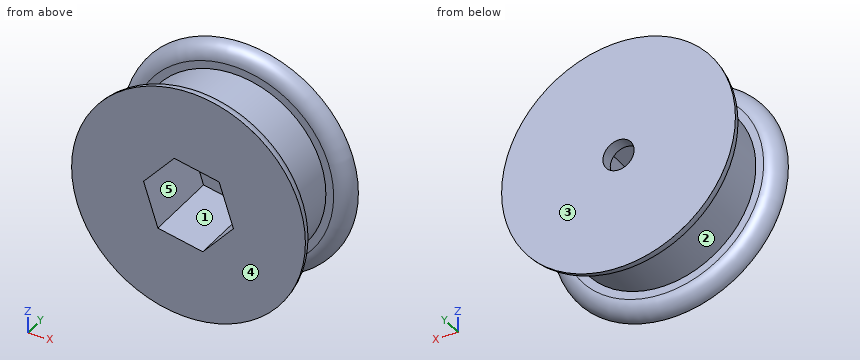
Autodesk Inventor part; units mm, degrees
ref_plane "YZ Plane" through (0, 0, 0) normal (1, 0, 0) x (0, 1, 0)
ref_plane "XZ Plane" through (0, 0, 0) normal (0, 1, 0) x (-1, 0, 0)
ref_plane "XY Plane" through (0, 0, 0) normal (0, 0, 1) x (1, 0, 0)
sketch "스케치1" plane through (0, 0, 0) normal (0, 1, 0) x (-1, 0, 0)
  line L0 (-0.9169, -2.7981) -> (-2.8817, -0.6049)
  line L1 (-2.8817, -0.6049) -> (-1.9647, 2.1931)
  line L2 (-1.9647, 2.1931) -> (0.9169, 2.7981)
  line L3 (0.9169, 2.7981) -> (2.8817, 0.6049)
  line L4 (2.8817, 0.6049) -> (1.9647, -2.1931)
  line L5 (1.9647, -2.1931) -> (-0.9169, -2.7981)
  circle A0 centre (0, 0) radius 7.5
  dimension "d0" = 5.1
  dimension "d1" = 15
extrude "돌출1" add sketch "스케치1" along normal blind 1
sketch "스케치2" plane through (0, 1, 0) normal (0, 1, 0) x (1, 0, 0)
  circle A0 centre (0, 0) radius 6
  line L0 (2.8817, 0.6049) -> (1.9647, -2.1931)
  line L1 (1.9647, -2.1931) -> (-0.9169, -2.7981)
  line L2 (-0.9169, -2.7981) -> (-2.8817, -0.6049)
  line L3 (-2.8817, -0.6049) -> (-1.9647, 2.1931)
  line L4 (-1.9647, 2.1931) -> (0.9169, 2.7981)
  line L5 (0.9169, 2.7981) -> (2.8817, 0.6049)
  circle A1 centre (0, 0) radius 7.5
  dimension "d4" = 12
extrude "돌출2" add sketch "스케치2" along normal blind 3.8 contours A0
sketch "스케치3" plane through (0, 4.8, 0) normal (0, 1, 0) x (1, 0, 0)
  circle A0 centre (0, 0) radius 7.5
  circle A1 centre (0, 0) radius 7.5
  line L0 (1.9647, -2.1931) -> (-0.9169, -2.7981)
  line L1 (-0.9169, -2.7981) -> (-2.8817, -0.6049)
  line L2 (-2.8817, -0.6049) -> (-1.9647, 2.1931)
  line L3 (-1.9647, 2.1931) -> (0.9169, 2.7981)
  line L4 (0.9169, 2.7981) -> (2.8817, 0.6049)
  line L5 (2.8817, 0.6049) -> (1.9647, -2.1931)
  circle A2 centre (0, 0) radius 6
  dimension "d7" = 15
extrude "돌출3" add sketch "스케치3" along normal blind 1 contours A0 | A2
sketch "스케치4" plane through (0, 5.8, 0) normal (0, 1, 0) x (1, 0, 0)
  point P0 (0, 0)
sketch "스케치5" plane through (0, 5.8, 0) normal (0, 1, 0) x (1, 0, 0)
  circle A0 centre (0, 0) radius 5
  circle A1 centre (0, 0) radius 1
  dimension "d10" = 10
  dimension "d11" = 2
extrude "돌출4" add sketch "스케치5" against normal blind 0.8
fillet "모깎기1" radius 1 2 edges at (7.5, 1, 0) (-7.5, 4.8, 0)
sketch "스케치6" plane through (0.9169, 0, -2.7981) normal (-0.7448, 0, 0.6673) x (0.6673, 0, 0.7448)
  point P0 (1.4722, 0)
sketch "스케치7" plane through (-2.8817, 0, 0.6049) normal (0.9503, 0, 0.3114) x (0.3114, 0, -0.9503)
  point P0 (1.4722, 0)
properties part number "motor gear"
Work out the finished part from the listing and answer in its coordinate system (mm). Face numbers are marked on the shaded views. A direction names the side the tool comes from. Round coordinates to 2 decimals unless told otherwise and drop trailing zeros. Order: outer loops, then holes, each group sorted by start corner. A loop starts at its lowest first (then second) coordinate and runs counter-clockwise, first axis right, second up. Notation, with made-up numbers: M 73.5,-4 L 100.5,-4 A15 cw 100.5,5 Z; hole C 17,25.5 d1. An arc over 180 degrees is marked long. Put each result on its own line as item: value. Start each with the question number.
Q1. Flat-ended cylindrical pins translate along their axes: pin 1 (3 mm diameter, centred on x = -2.5, y = 3, fed in from -Z); pin 2 (2 mm diameter, centred on x = 0, y = 2.5, fed in from +Z); pin 3 (4 mm diameter, centred on x = 0, z = 0.5, fed in from -Y). Find the tip coordinate at first contact, or state that the pin passes through.
Q2. Straight lines are drawn through the part: L1, parallel to Y at x = -6, z = 1.25; L2, parallel to X at y = 2, z = 1; L3, parallel to Y at x = -1.25, z = -1.5. For each, find the intervals that lie inside material, in ascending order. Write a range as [from, to].
Q3. Section A-A, the plane y = 2.1 is taken. Write down the section's boundary in (x, z), and give its area (3 significant figures).
Q4. For a pull along X with two mould halves and no side action, classify the marked faces 1, 2 and 3 as pulls with the +X half, pulls with the -X half, needs draft (parallel to the pull), parting line crosses it, or undercut.
Q5. A tool of negligible diameter and unlimited length cuts with its end or side. For the marked faces 4 and 5, from which of +Z, -Z, +X, -X, +Y, -Y can it reach the whole face along a straight path? Write none if from no direction.
Findings below:
1. pin 1: stops at z = -5.92
1. pin 2: stops at z = 6
1. pin 3: stops at y = 5
2. L1: y = [0, 1], [4.8, 5.8]
2. L2: x = [-5.92, -2.53], [2.36, 5.92]
2. L3: y = [5, 5.8]
3. outline: C 0,0 d12; hole M -2.88,0.6 L -1.96,-2.19 L 0.92,-2.8 L 2.88,-0.6 L 1.96,2.19 L -0.92,2.8 Z
3. area: 90.6 mm^2
4. face 1: undercut
4. face 2: parting line crosses it
4. face 3: needs draft
5. face 4: +Z, -Z, +X, -X, -Y
5. face 5: -Y
